Geometry check sheet. Reference: the model listing, model coordinates, mm. Coordinates: 2 decimals unless noted, no trailing zeros. Order: outer loops, then holes, each group sorted by start corner. A loop starts at its lowest first (then second) coordinate and runs counter-clockwise, first axis right, second up.
```python
from build123d import *

# Parameters (mm, degrees)
SKETCH1_W             = 150
SKETCH1_H             = 400
BOSS_EXTRUDE1_DEPTH   = 3
SKETCH6_R             = 4.232555097
CUT_EXTRUDE5_DEPTH    = 3
CAVITY1_START         = -75
CAVITY1_OUTLINE_W     = 50
CAVITY1_OUTLINE_H     = 3
CAVITY1_OUTLINE_W_2   = 47
CAVITY1_OUTLINE_W_3   = 25
CAVITY1_DEPTH         = 3
CAVITY1_START_2       = 72
CAVITY1_2_OUTLINE_W   = 50
CAVITY1_2_OUTLINE_H   = 3
CAVITY1_2_OUTLINE_W_2 = 47
CAVITY1_2_OUTLINE_W_3 = 25
CAVITY1_2_DEPTH       = 3
CAVITY1_START_3       = -55
CAVITY1_3_OUTLINE_W   = 3
CAVITY1_3_OUTLINE_H   = 3
CAVITY1_3_DEPTH       = 110
SKETCH7_W             = 107.112189612
SKETCH7_H             = 234.735224044
CUT_EXTRUDE6_DEPTH    = 10


# Read off the part's stored shape, not the designer's step: Cavity1
with BuildPart() as part:
    # Sketch1 → Boss-Extrude1 (new body)
    with BuildSketch(Plane.XY):
        Rectangle(SKETCH1_W, SKETCH1_H)
    extrude(amount=BOSS_EXTRUDE1_DEPTH)

    # Sketch6 → Cut-Extrude5 (cut)
    with BuildSketch(Plane(origin=(0, 0, 0), x_dir=(-1, 0, 0), z_dir=(0, 0, -1))):
        with Locations((-2.75, -138.3)):
            Circle(SKETCH6_R)
    extrude(amount=-CUT_EXTRUDE5_DEPTH, mode=Mode.SUBTRACT)

    # Cavity1 outline → Cavity1 (cut)
    with BuildSketch(Plane.YZ.offset(CAVITY1_START)):
        with Locations((122, 1.5)):
            Rectangle(CAVITY1_OUTLINE_W, CAVITY1_OUTLINE_H)
        with Locations((23.5, 1.5)):
            Rectangle(CAVITY1_OUTLINE_W_2, CAVITY1_OUTLINE_H)
        with Locations((-62.5, 1.5)):
            Rectangle(CAVITY1_OUTLINE_W_3, CAVITY1_OUTLINE_H)
        with Locations((-137.5, 1.5)):
            Rectangle(CAVITY1_OUTLINE_W_3, CAVITY1_OUTLINE_H)
    extrude(amount=CAVITY1_DEPTH, mode=Mode.SUBTRACT)

    # Cavity1 2 outline → Cavity1 2 (cut)
    with BuildSketch(Plane.YZ.offset(CAVITY1_START_2)):
        with Locations((122, 1.5)):
            Rectangle(CAVITY1_2_OUTLINE_W, CAVITY1_2_OUTLINE_H)
        with Locations((23.5, 1.5)):
            Rectangle(CAVITY1_2_OUTLINE_W_2, CAVITY1_2_OUTLINE_H)
        with Locations((-62.5, 1.5)):
            Rectangle(CAVITY1_2_OUTLINE_W_3, CAVITY1_2_OUTLINE_H)
        with Locations((-137.5, 1.5)):
            Rectangle(CAVITY1_2_OUTLINE_W_3, CAVITY1_2_OUTLINE_H)
    extrude(amount=CAVITY1_2_DEPTH, mode=Mode.SUBTRACT)

    # Cavity1 3 outline → Cavity1 3 (cut)
    with BuildSketch(Plane.YZ.offset(CAVITY1_START_3)):
        with Locations((-99.307385879, 1.5)):
            Rectangle(CAVITY1_3_OUTLINE_W, CAVITY1_3_OUTLINE_H)
    extrude(amount=CAVITY1_3_DEPTH, mode=Mode.SUBTRACT)

    # Sketch7 → Cut-Extrude6 (cut)
    with BuildSketch(Plane.XY.offset(3)):
        with Locations((0, 54.41071334)):
            Rectangle(SKETCH7_W, SKETCH7_H)
    extrude(amount=-CUT_EXTRUDE6_DEPTH, mode=Mode.SUBTRACT)


solid = part.part
```
Item 1: Sectioned sample at A-A (y = 14). Record the cut outline in (x, z).
Item 2: Sectioned sample at B-B (x = 17.5). Record the cut outline in (y, z).
Item 3: Release check for a two-part mould opening along Y. For faces 1 (the face through (0.475, -134.731, 1.479)), 2 (the face through (-1, -86, 3)) record: pulls with the +Y half, pulls with the -Y half, needs draft (parallel to the pull), parting line crosses it, or undercut.
Item 4: Thickness scan on line 1 along Y through (x, z) = (-20, 2.35); line 2 along Y through (x, z) = (2.75, 1.3); line 3 along X through (y, z) = (43, 2.3). Record the ranges inside material, lowest first.
Item 5: Sectioned sample at D-D (z = 1.4). Give the number of separate pieces and of enclosed holes in the cut face, and give its area (3 significant figures).
Item 6: Depth check by flat-ended pin: P1, Ø1.5, axis at y = 125, z = 1, coming from the +X side. Enter the tip coordinate at first touch or a pass-through.
Item 7: Sectioned sample at C-C (y = 88.5). Record the cut outline in (x, z).
Geometry check:
1. outline: (-72, 0) - (-53.56, 0) - (-53.56, 3) - (-72, 3) - close; (53.56, 0) - (72, 0) - (72, 3) - (53.56, 3) - close
2. outline: (-200, 0) - (-100.81, 0) - (-100.81, 3) - (-200, 3) - close; (-97.81, 0) - (-62.96, 0) - (-62.96, 3) - (-97.81, 3) - close; (171.78, 0) - (200, 0) - (200, 3) - (171.78, 3) - close
3. face 1: undercut
3. face 2: needs draft
4. line 1: y = -200 to -100.81, -97.81 to -62.96, 171.78 to 200
4. line 2: y = -200 to -142.53, -134.07 to -100.81, -97.81 to -62.96, 171.78 to 200
4. line 3: x = -72 to -53.56, 53.56 to 72
5. separate pieces: 1
5. enclosed holes: 3
5. area: 33,600 mm2
6. P1: stops at x = 72
7. outline: (-75, 0) - (-53.56, 0) - (-53.56, 3) - (-75, 3) - close; (53.56, 0) - (75, 0) - (75, 3) - (53.56, 3) - close
